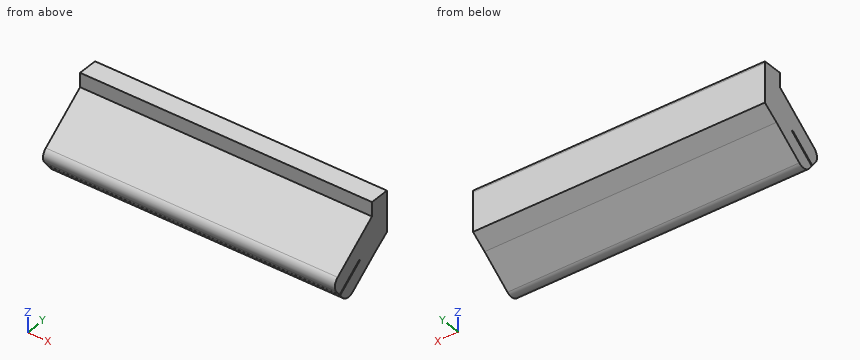
from build123d import *

# Parameters (mm, degrees)
F1_DEPTH = 120.523
F2_R     = 3.81


with BuildPart() as f1:
    # F0 (on Right) → F1 (new body)
    with BuildSketch(Plane.YZ):
        Polygon((8.171235, 5.354634), (0, 16.249614), (-21.666151, 0), (-17.617675, -5.397966), (-6.796981, 2.717555), (-6.470074, 2.281679), (-17.229717, -5.788053), (-13.594393, -10.63515), (1.864555, 0.959061), align=None)
        Polygon((0, 22.087431), (0, 16.249614), (8.171235, 5.354634), (8.171235, 21.347754), (8.125494, 22.087431), align=None)
    extrude(amount=F1_DEPTH)

    # F2
    f2_edges = [f1.edges().sort_by_distance(p)[0] for p in [
        (60.2615, -21.666151, 0),
        (60.2615, -13.594393, -10.63515),
    ]]
    fillet(f2_edges, radius=F2_R)


solid = f1.part
Could you check a few things on this model? Use its own coordinates, in mm. Give positions to 0.01 mm unless a question says otherwise; leave off trailing zeros. Write each loop counter-clockwise with the first axis right and the second up, starting at its lowest first coordinate (ties: lowest second). Pieces come first, ordered by that corner, then holes. Notation, with made-up numbers: (41, -16.5) - (75, -16.5) arc R17 cw to (75, 16.5) - close; hole circle Ø6 at (41.5, 30). An arc over 180 degrees is marked (long way). Use CSV: the item, a comma, the result in double quotes. Start each with the question number.
Item 1: If I drill on line 1 along Z through (x, y) = (90.5, -9); line 2 along Y through (x, z) = (98, 10); line 3 along Y through (x, z) = (58, 2.5), over which ranges is the centre line in solid material (lowest first)?
Item 2: I want a section at C-C, the plane y = -3.5. Please give me the cut outline in (x, z).
Item 3: I'm going to push flat-ended pins straight in: pin 1 (4 mm diameter, centred on x = 20, y = -15, fed in from +Z); pin 2 (2 mm diameter, centred on x = 84, z = -3, fed in from +Y); pin 3 (4 mm diameter, centred on x = 72, y = -13, fed in from +Z). Where does each tip first touch, or does it pass through?
Item 4: I want a section at A-A, the plane x = 103. Please give me the cut outline in (y, z), then the cut area to 3 significant figures.
Item 5: I want a section at B-B, the plane z = 13.5. Please give me the cut outline in (x, y), then the cut area to 3 significant figures.
Findings:
1,line 1,"z = -7.19 to 0.38, 1.07 to 9.5"
1,line 2,"y = -8.33 to 8.17"
1,line 3,"y = -18.33 to -7.09, -6.63 to 4.08"
2,outline,"(0, -3.06) - (120.52, -3.06) - (120.52, 13.62) - (0, 13.62) - close"
3,pin 1,"stops at z = 6.5"
3,pin 2,"stops at y = -2.08"
3,pin 3,"stops at z = 8"
4,outline,"(-19.38, -3.05) - (-17.62, -5.4) - (-6.8, 2.72) - (-6.47, 2.28) - (-17.23, -5.79) - (-15.88, -7.59) arc R3.81 ccw to (-10.55, -8.35) - (1.86, 0.96) - (8.17, 5.35) - (8.17, 21.35) - (8.13, 22.09) - (0, 22.09) - (0, 16.25) - (-18.62, 2.29) arc R3.81 ccw to start"
4,area,"441 mm2"
5,outline,"(0, -3.67) - (120.52, -3.67) - (120.52, 8.17) - (0, 8.17) - close"
5,area,"1,430 mm2"
